Check sheet for the drawn part. Datum: minimum x, y, z corner. Units: mm. A direction names the side the tool comes from. Give positions to 0.01 mm unless a question says otherwise; leave off trailing zeros. Write each loop counter-clockwise with the first axis right and the second up, starting at its lowest first coordinate (ties: lowest second). Pieces come first, ordered by that corner, then holes. Notation, with made-up numbers: (-19.5, -27.5) -> (-8.5, -27.5) arc R33 ccw to (-8.5, 2.5) -> close; hole circle Ø2 at (23.25, 44). An arc over 180 degrees is marked (long way). Write item = value, one per line. Start each with the question number.
1. Cross-section at B-B, the plane z = 13. Record the cut outline in (x, y), plus the area to 3 significant figures.
2. Set-up check for the marked faces 3 and 4: record each of +Z, -Z, +X, -X, +Y, -Y from which the full face is reachable in a straight line by a thin tool's end or side.
3. Mould release check, pull along Y, two halves, no side actions. Record for the marked faces 1 and 2: pulls with the +Y half, pulls with the -Y half, needs draft (parallel to the pull), parting line crosses it, or undercut.
4. Thickness scan on line 1 along X through (y, z) = (47, 10); line 2 along Y through (x, z) = (47, 5). Record the ranges inside material, lowest first.
5. Cross-section at A-A, the plane z = 23. Record the cut outline in (x, y), plus the area to 3 significant figures.
6. Depth check by flat-ended pin: P1, Ø10, axis at y = 20, z = 22.5, coming from the +X side (1 decimal); P2, Ø6, axis at x = 71, z = 8, coming from the +Y side; P3, Ø2, axis at x = 53, y = 74, coming from the +Z side. Enter the tip coordinate at first touch or a pass-through.
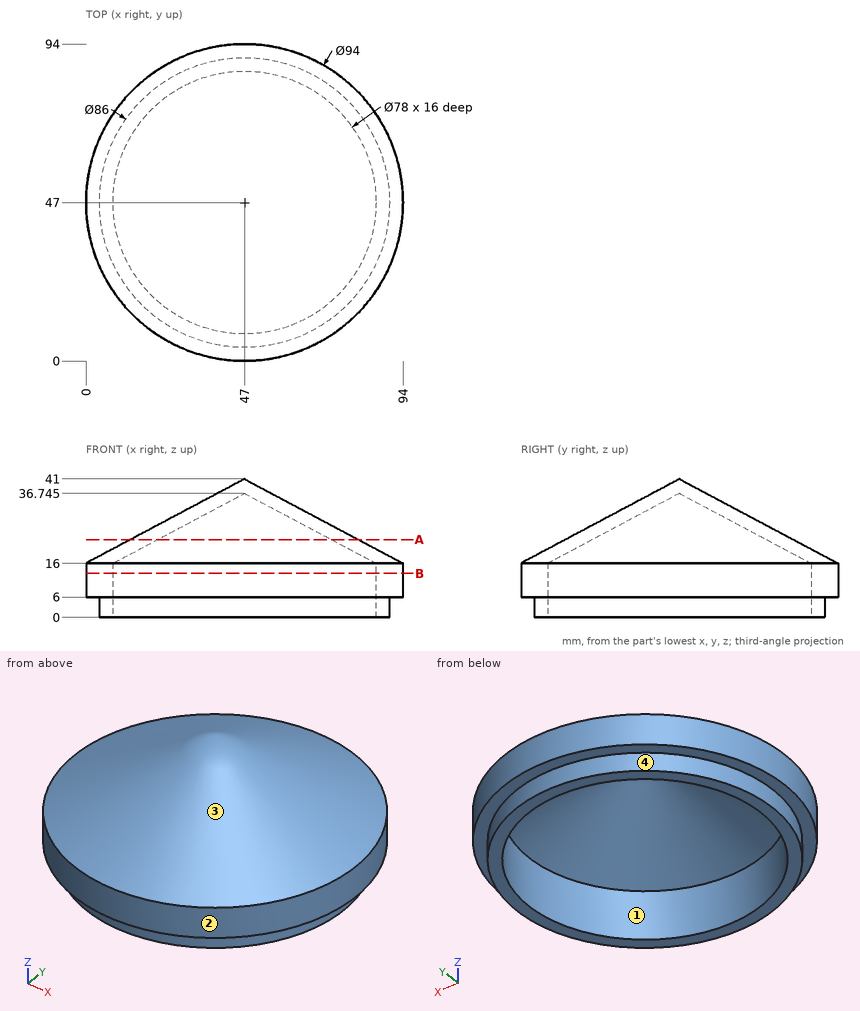
Answers:
q1.outline = circle Ø94 at (47, 47); hole circle Ø78 at (47, 47)
q1.area = 2,160 mm^2
q2.face_3 = +Z
q2.face_4 = -Z
q3.face_1 = undercut
q3.face_2 = parting line crosses it
q4.line_1 = 0 to 8, 86 to 94
q4.line_2 = 4 to 8, 86 to 90
q5.outline = circle Ø67.68 at (47, 47); hole circle Ø51.68 at (47, 47)
q5.area = 1,500 mm^2
q6.P1 = 82.5
q6.P2 = 89.05
q6.P3 = 26.82
